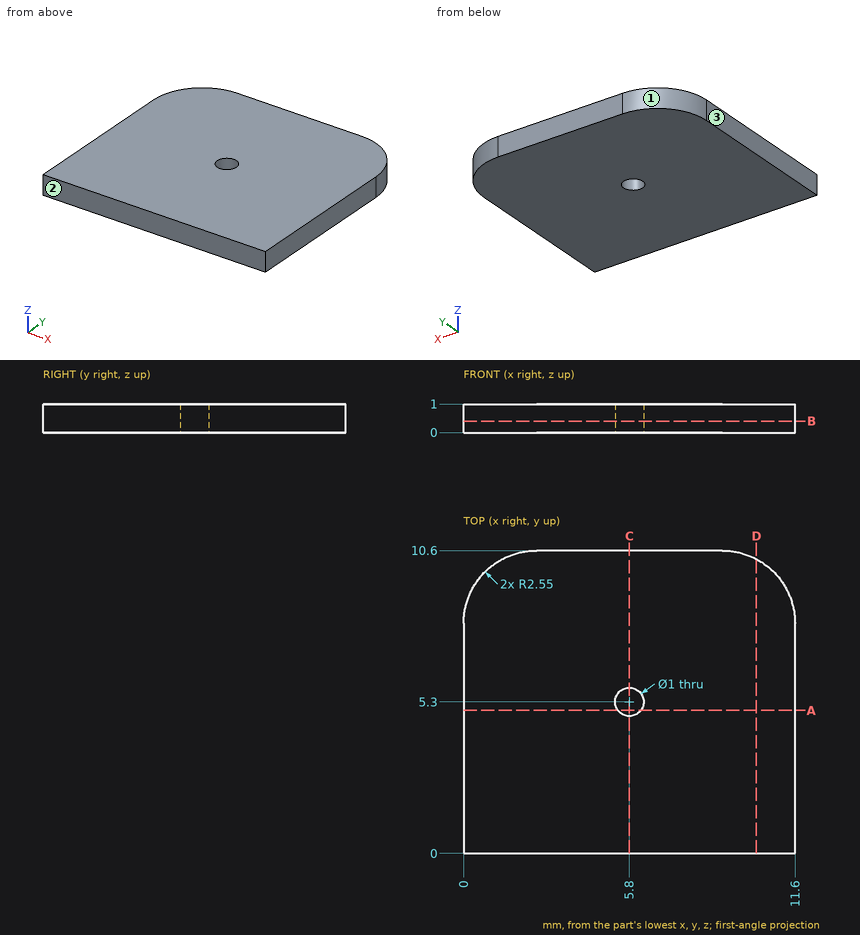
Could you check a few things on this drawing? It's one solid part, dimensions in mm from its lowest x, y, z. Give positions to 0.01 mm unless a question says otherwise; leave off trailing zeros. Loops run counter-clockwise (first coordinate to the right, second up) from the corner with the lowest first, then second, coordinate; pieces in that order, holes last. Notation, with made-up numbers: (-7.75, -7) -> (11.25, -7) arc R23 ccw to (11.25, 29) -> close; hole circle Ø1 at (-35, 75). An arc over 180 degrees is marked (long way). Use one line per item in the form item = value. Start each with the question number.
1) For P1, Ø1, axis at x = 8.5, y = 4, coming from the -Z side, with a flat end and sliding along its axis, tell me the tip position at first contact or that it passes through.
2) Imagine slicing it at A-A (y = 5). Please give me the cut outline in (x, z).
3) Thinking about a two-plate mould opening in Y: for the marked faces 1, 2 and 3, which applies, +Y half, -Y half, draft (parallel to the pull), parting line (faces both ways), or undercut?
4) Imagine slicing it at C-C (x = 5.8). Please give me the cut outline in (y, z), then the cut area to 3 significant figures.
5) Please list where these lines run through material, in increasing order: line 1 along Y through (x, z) = (5.8, 0.3); line 2 along X through (y, z) = (5.3, 0.3); line 3 along X through (y, z) = (10.25, 0.7).
6) Imagine slicing it at B-B (z = 0.4). Please give me the cut outline in (x, y), then the cut area to 3 significant figures.
7) Imagine slicing it at D-D (x = 10.25). Please give me the cut outline in (y, z).
Check values:
q1.P1 = 0
q2.outline = (0, 0) -> (5.4, 0) -> (5.4, 1) -> (0, 1) -> close; (6.2, 0) -> (11.6, 0) -> (11.6, 1) -> (6.2, 1) -> close
q3.face_1 = +Y half
q3.face_2 = -Y half
q3.face_3 = draft
q4.outline = (0, 0) -> (4.8, 0) -> (4.8, 1) -> (0, 1) -> close; (5.8, 0) -> (10.6, 0) -> (10.6, 1) -> (5.8, 1) -> close
q4.area = 9.60 mm^2
q5.line_1 = 0 to 4.8, 5.8 to 10.6
q5.line_2 = 0 to 5.3, 6.3 to 11.6
q5.line_3 = 1.26 to 10.34
q6.outline = (0, 0) -> (11.6, 0) -> (11.6, 8.05) arc R2.55 ccw to (9.05, 10.6) -> (2.55, 10.6) arc R2.55 ccw to (0, 8.05) -> close; hole circle Ø1 at (5.8, 5.3)
q6.area = 119 mm^2
q7.outline = (0, 0) -> (10.3, 0) -> (10.3, 1) -> (0, 1) -> close
